Can you work these out from the model? Positions are in its coordinate system, mm. A direction names the side the tool comes from. Give positions to 0.01 mm unless a question says otherwise; leave off trailing zeros.
Item 1: If I drill on line 1 along Y through (x, z) = (0, 2.25); line 2 along Z through (x, y) = (28.5, -16); line 3 along X through (y, z) = (7.5, 3), over which ranges is the centre line in solid material (lowest first)?
Item 2: I'm going to push flat-ended pins straight in: pin 1 Ø3.5 at (x, y) = (-3.5, 33) entering from +Z; pin 2 Ø2 at (x, z) = (-13.5, -2.5) entering from +Y; pin 3 Ø2 at (x, y) = (3.5, -33.5) entering from -Z; pin 4 Ø2 at (x, z) = (-3.5, 0.5) entering from -Y. Where does each tip first touch, or does it pass through?
Item 3: Which directions (+Z, -Z, +X, -X, +Y, -Y) give clear straight access to the entire face, cutting with the end or side of a thin tool? Please do faces 1 (the cylindrical face through (14.9, 28.6, -2.6)), 2 (the flat face through (29, -17, 2)), 3 (the cylindrical face through (-2.55, -38.58, 0.03)), 4 (the cylindrical face through (-2.596, 38.467, 0.028)).
Item 4: If we mould it in two halves opening along Y, with no side actions, what happens to faces 5 (the cylindrical face through (34.7, 17.1, 0)), 6 (the cylindrical face through (38.467, 2.596, 0.028)), 7 (the flat face through (-17, -29, 2)), 8 (the cylindrical face through (-32.136, 21.496, 0.028))? For each: +Y half, -Y half, draft (parallel to the pull), parting line (faces both ways), or undercut.
```python
from build123d import *

# Parameters (mm, degrees)
EXTRUDE_1_DEPTH          = 2
CUT_EXTRUDE_1_DEPTH      = 6
PATTERN_CIRCULAR_1_COUNT = 12
SKETCH_6_R               = 32.25
SKETCH_6_R_2             = 10
EXTRUDE_2_DEPTH          = 3.5
FILLET_1_R               = 0.35


with BuildPart() as part:
    # Sketch 4 → Extrude 1 (new, symmetric)
    with BuildSketch(Plane.XY):
        with BuildLine():
            Line((-0.25, 43.320508076), (0.25, 43.320508076))
            ThreePointArc((0.25, 43.320508076), (2.185336575, 39.411779528), (3.8, 35.360045512))
            ThreePointArc((3.8, 35.360045512), (5.552858836, 32.693174534), (8.346914205, 31.151107898))
            ThreePointArc((8.346914205, 31.151107898), (0, 32.25), (-8.346914205, 31.151107898))
            ThreePointArc((-8.346914205, 31.151107898), (-5.552858836, 32.693174534), (-3.8, 35.360045512))
            ThreePointArc((-3.8, 35.360045512), (-2.185336575, 39.411779528), (-0.25, 43.320508076))
        make_face()
    extrude(amount=EXTRUDE_1_DEPTH, both=True)

    # Sketch 5 → Cut-Extrude 1 (cut, symmetric)
    with BuildSketch(Plane(origin=(0, 0, 0), x_dir=(0, 0, -1), z_dir=(1, 0, 0))):
        with BuildLine():
            Line((-2, 35.360045512), (-3, 35.360045512))
            Line((-3, 35.360045512), (-3, 44.320508076))
            Line((-3, 44.320508076), (3, 44.320508076))
            Line((3, 44.320508076), (3, 35.360045512))
            Line((3, 35.360045512), (2, 35.360045512))
            ThreePointArc((2, 35.360045512), (1.451594964, 39.412074278), (0.25, 43.320508076))
            Line((0.25, 43.320508076), (-0.25, 43.320508076))
            ThreePointArc((-0.25, 43.320508076), (-1.451594964, 39.412074278), (-2, 35.360045512))
        make_face()
    extrude(amount=CUT_EXTRUDE_1_DEPTH, both=True, mode=Mode.SUBTRACT)


with BuildPart() as pattern_circular_1_1:
    # Pattern Circular 1: pattern copy
    add(part.part.rotate(Axis((0, 0, 0), (0, 0, 1)), 1 * 360 / PATTERN_CIRCULAR_1_COUNT))


with BuildPart() as pattern_circular_1_2:
    # Pattern Circular 1: pattern copy
    add(part.part.rotate(Axis((0, 0, 0), (0, 0, 1)), 2 * 360 / PATTERN_CIRCULAR_1_COUNT))


with BuildPart() as pattern_circular_1_3:
    # Pattern Circular 1: pattern copy
    add(part.part.rotate(Axis((0, 0, 0), (0, 0, 1)), 3 * 360 / PATTERN_CIRCULAR_1_COUNT))


with BuildPart() as pattern_circular_1_4:
    # Pattern Circular 1: pattern copy
    add(part.part.rotate(Axis((0, 0, 0), (0, 0, 1)), 4 * 360 / PATTERN_CIRCULAR_1_COUNT))


with BuildPart() as pattern_circular_1_5:
    # Pattern Circular 1: pattern copy
    add(part.part.rotate(Axis((0, 0, 0), (0, 0, 1)), 5 * 360 / PATTERN_CIRCULAR_1_COUNT))


with BuildPart() as pattern_circular_1_6:
    # Pattern Circular 1: pattern copy
    add(part.part.rotate(Axis((0, 0, 0), (0, 0, 1)), 6 * 360 / PATTERN_CIRCULAR_1_COUNT))


with BuildPart() as pattern_circular_1_7:
    # Pattern Circular 1: pattern copy
    add(part.part.rotate(Axis((0, 0, 0), (0, 0, 1)), 7 * 360 / PATTERN_CIRCULAR_1_COUNT))


with BuildPart() as pattern_circular_1_8:
    # Pattern Circular 1: pattern copy
    add(part.part.rotate(Axis((0, 0, 0), (0, 0, 1)), 8 * 360 / PATTERN_CIRCULAR_1_COUNT))


with BuildPart() as pattern_circular_1_9:
    # Pattern Circular 1: pattern copy
    add(part.part.rotate(Axis((0, 0, 0), (0, 0, 1)), 9 * 360 / PATTERN_CIRCULAR_1_COUNT))


with BuildPart() as pattern_circular_1_10:
    # Pattern Circular 1: pattern copy
    add(part.part.rotate(Axis((0, 0, 0), (0, 0, 1)), 10 * 360 / PATTERN_CIRCULAR_1_COUNT))


with BuildPart() as pattern_circular_1_11:
    # Pattern Circular 1: pattern copy
    add(part.part.rotate(Axis((0, 0, 0), (0, 0, 1)), 11 * 360 / PATTERN_CIRCULAR_1_COUNT))


with BuildPart() as part_1:
    add(part.part)

    add(pattern_circular_1_1.part)  # Extrude 2 merges Pattern Circular 1_1

    add(pattern_circular_1_2.part)  # Extrude 2 merges Pattern Circular 1_2

    add(pattern_circular_1_3.part)  # Extrude 2 merges Pattern Circular 1_3

    add(pattern_circular_1_4.part)  # Extrude 2 merges Pattern Circular 1_4

    add(pattern_circular_1_5.part)  # Extrude 2 merges Pattern Circular 1_5

    add(pattern_circular_1_6.part)  # Extrude 2 merges Pattern Circular 1_6

    add(pattern_circular_1_7.part)  # Extrude 2 merges Pattern Circular 1_7

    add(pattern_circular_1_8.part)  # Extrude 2 merges Pattern Circular 1_8

    add(pattern_circular_1_9.part)  # Extrude 2 merges Pattern Circular 1_9

    add(pattern_circular_1_10.part)  # Extrude 2 merges Pattern Circular 1_10

    add(pattern_circular_1_11.part)  # Extrude 2 merges Pattern Circular 1_11
    # Sketch 6 → Extrude 2 (add, symmetric)
    with BuildSketch(Plane.XY):
        with Locations(Location((0, 0, 0), (0, 0, 165))):
            Circle(SKETCH_6_R)
        Circle(SKETCH_6_R_2, mode=Mode.SUBTRACT)
    extrude(amount=EXTRUDE_2_DEPTH, both=True)

    # Fillet 1
    fillet_1_edges = [part_1.edges().sort_by_distance(p)[0] for p in [
        (31.151107898, -8.346914205, 3.5),
        (31.151107898, -8.346914205, -3.5),
    ]]
    fillet(fillet_1_edges, radius=FILLET_1_R)


solid = part_1.part
```
Results list:
1. line 1: y = -32.25 to -10, 10 to 32.25
1. line 2: z = -2 to 2
1. line 3: x = -31.37 to -6.61, 6.61 to 31.37
2. pin 1: stops at z = 3.5
2. pin 2: stops at y = 32.5
2. pin 3: stops at z = -2
2. pin 4: stops at y = -38.69
3. face 1: -Z
3. face 2: +Z, +X, -Y
3. face 3: +Z, -Z, -Y
3. face 4: +Z, -Z, +Y
4. face 5: undercut
4. face 6: undercut
4. face 7: draft
4. face 8: +Y half
